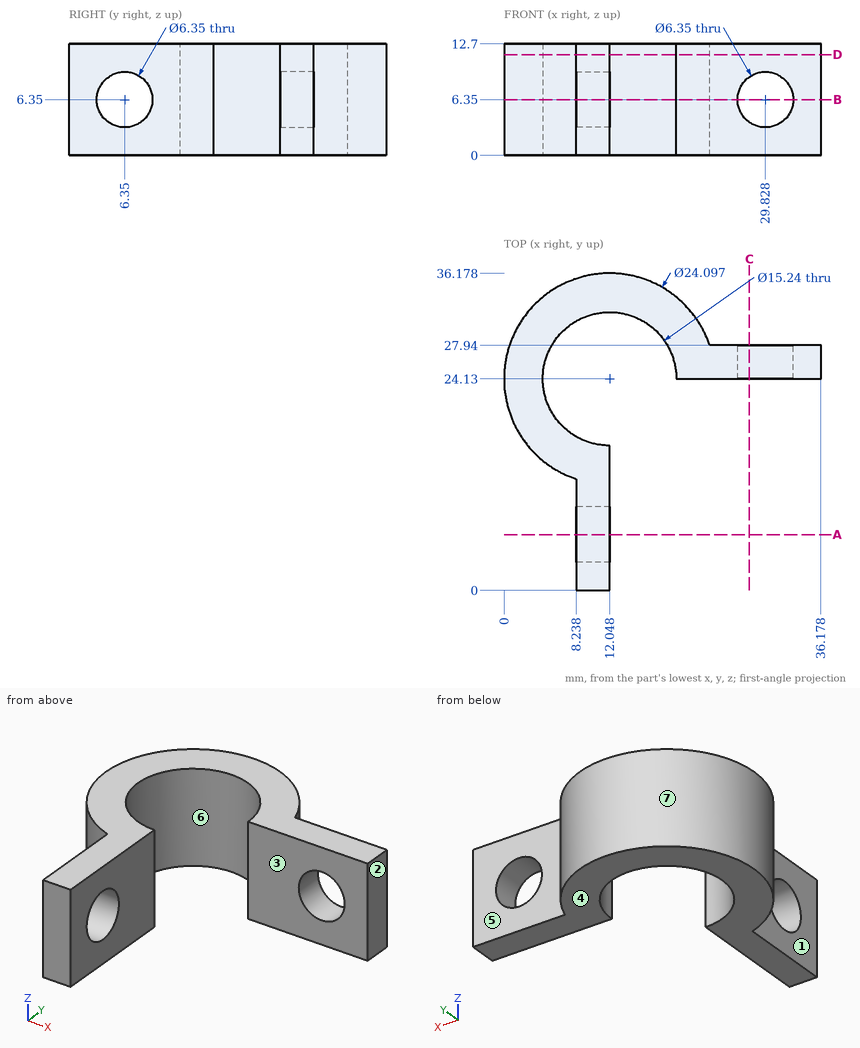
The figure shows three views and two pictorial views of one solid part (mm, origin at its lowest corner). Answer the questions. A direction names the side the tool comes from. Round coordinates to 2 decimals unless told otherwise and drop trailing zeros. Loops run counter-clockwise (first coordinate to the right, second up) from the corner with the lowest first, then second, coordinate; pieces in that order, holes last. Notation, with made-up numbers: M 56.25,85 L 83.25,85 A4 ccw 83.25,89 Z; hole C 42,40 d5. An arc over 180 degrees is marked long. Write each question's results on one line, items separated by ' | '. Start each with the question number.
1) Which of the six approach directions +Z, -Z, +X, -X, +Y, -Y give full straight-line access (tool end or side, diameter ignored) to the marked faces 1, 2 and 3?
2) Find section C-C on x = 28. Write down the section's boundary in (y, z) (1 decimal), plus the area to 3 significant figures.
3) Determine the mould class of the marked faces 4, 5, 6 and 7 for opening direction Y: pulls with the +Y half, pulls with the -Y half, needs draft (parallel to the pull), parting line crosses it, or undercut.
4) Find section A-A on y = 6.35. Write down the section's boundary in (x, z) (1 decimal).
5) Each of these flat-tipped pins is pushed along its axis until it touches: pin 1 (1.5 mm diameter, centred on y = 21, z = 9.5, fed in from +X); pin 2 (1.5 mm diameter, centred on x = 30, z = 11, fed in from -Y); pin 3 (6.5 mm diameter, centred on y = 4, z = 6, fed in from +X); pin 4 (9 mm diameter, centred on x = 12.05, y = 24.13, fed in from -Z). Where does it stop, or does it pass through?
6) Find section B-B on z = 6.35. Write down the section's boundary in (x, y) (1 decimal).
7) Straight lines are drawn through the part: probe 1 along Y at (x, z) = (9.05, 6.35) (1 decimal); probe 2 along Y at (x, z) = (12, 5.75); probe 3 along X at (y, z) = (3, 10.5). For each, find the intervals that lie inside material, in ascending order.
8) Find section D-D on z = 11.5. Write down the section's boundary in (x, y).
Final values:
1) face 1: +Z, -Z, -X, -Y | face 2: +Z, -Z, +X, +Y, -Y | face 3: +Z, -Z, +X, -Y
2) outline: M 24.1,0 L 27.9,0 L 27.9,3.8 L 24.1,3.8 Z; M 24.1,8.9 L 27.9,8.9 L 27.9,12.7 L 24.1,12.7 Z | area: 28.6 mm²
3) face 4: needs draft | face 5: pulls with the +Y half | face 6: undercut | face 7: parting line crosses it
4) outline: M 8.2,0 L 12,0 L 12,3.2 L 8.2,3.2 Z; M 8.2,9.5 L 12,9.5 L 12,12.7 L 8.2,12.7 Z
5) pin 1: x = 5.49 | pin 2: y = 24.13 | pin 3: x = 12.05 | pin 4: through
6) outline: M 8.2,0 L 12,0 L 12,3.2 L 8.2,3.2 Z; M 8.2,9.5 L 12,9.5 L 12,16.5 A7.6 cw long 19.7,24.1 L 26.7,24.1 L 26.7,27.9 L 23.5,27.9 A12 ccw long 8.2,12.7 Z; M 33,24.1 L 36.2,24.1 L 36.2,27.9 L 33,27.9 Z
7) probe 1: 0 to 3.2, 9.5 to 17.1, 31.1 to 35.8 | probe 2: 0 to 3.23, 9.47 to 16.51, 31.75 to 36.18 | probe 3: 8.24 to 12.05
8) outline: M 8.24,0 L 12.05,0 L 12.05,16.51 A7.62 cw long 19.67,24.13 L 36.18,24.13 L 36.18,27.94 L 23.48,27.94 A12.05 ccw long 8.24,12.7 Z
